from build123d import *

# Parameters (mm, degrees)
BOSS_EXTRUDE1_DEPTH = 1500
FILLET1_R           = 10
SKETCH2_R           = 37.5
CUT_EXTRUDE1_DEPTH  = 1540.683409016


with BuildPart() as part:
    # Sketch1 → Boss-Extrude1 (new body)
    with BuildSketch(Plane(origin=(0, 0, 0), x_dir=(1, 0, 0), z_dir=(0, 1, 0))):
        Polygon((175, 50), (300, 50), (300, 0), (0, 0), (0, 50), (125, 50), (125, 250), (0, 250), (0, 300), (300, 300), (300, 250), (175, 250), align=None)
    extrude(amount=BOSS_EXTRUDE1_DEPTH)

    # Fillet1
    fillet1_edges = [part.edges().sort_by_distance(p)[0] for p in [
        (125, 750, -50),
        (125, 750, -250),
        (175, 750, -250),
        (175, 750, -50),
    ]]
    fillet(fillet1_edges, radius=FILLET1_R)

    # Sketch2 → Cut-Extrude1 (cut, through all)
    with BuildSketch(Plane.ZY.offset(-125)):
        with Locations((-150, 1400)):
            Circle(SKETCH2_R)
        with Locations((-150, 1000)):
            Circle(SKETCH2_R)
    extrude(amount=-CUT_EXTRUDE1_DEPTH, mode=Mode.SUBTRACT)


solid = part.part
Read the model definition and answer for the solid it produces. Units are mm, in the model's axes. A direction names the side the tool comes from. Round coordinates to 2 decimals unless told otherwise and drop trailing zeros. Order: outer loops, then holes, each group sorted by start corner. A loop starts at its lowest first (then second) coordinate and runs counter-clockwise, first axis right, second up. Notation, with made-up numbers: (-15, 27.5) - (38, 27.5) arc R11 cw to (38, 33.5) - close; hole circle Ø11 at (7.25, 21.5). An arc over 180 degrees is marked (long way). Use one line per item in the form item = value. Start each with the question number.
(1) The part is cut by section D-D (y = 580). Give the vertices of the cut face in (x, z).
(2) Determine the mould class of faces 1 (the face through (152, 1500, -185)), 2 (the face through (242, 740, -50)), 3 (the face through (149.65, 966.73, -132.7)) for opening direction Y: +Y half, -Y half, draft (parallel to the pull), parting line (faces both ways), or undercut.
(3) For faces 4 (the face through (58, 740, -250)), 5 (the face through (0, 740, -275)), 6 (the face through (175, 740, -151)), determine the directions among +Z, -Z, +X, -X, +Y, -Y from which every point of the face is accessible in a straight line to the end or side of a thin tool.
(4) The part is cut by section C-C (z = -150). Give the vertices of the cut face in (x, y), then the cut area to 3 significant figures.
(5) The part is cut by section A-A (x = 262). Give the vertices of the cut face in (y, z).
(6) Flat-ended cylindrical pins translate along their axes: pin 1 Ø6 at (y, z) = (675.5, -171) entering from +X; pin 2 Ø6 at (y, z) = (1156, -55.5) entering from -X. Find the tip coordinate at first contact, or state that the pin passes through.
(7) The part is cut by section B-B (y = 1000). Give the vertices of the cut face in (x, z), then the cut area to 3 significant figures.
(8) Find the intervals of material crossed by line 1 along Y through (x, z) = (140, -150); line 2 along Z through (x, y) = (282.5, 388); line 3 along X through (y, z) = (1359, -98), in increasing order. Write a range as from..to.
Checked values:
q1.outline = (0, -300) - (300, -300) - (300, -250) - (185, -250) arc R10 cw to (175, -240) - (175, -60) arc R10 cw to (185, -50) - (300, -50) - (300, 0) - (0, 0) - (0, -50) - (115, -50) arc R10 cw to (125, -60) - (125, -240) arc R10 cw to (115, -250) - (0, -250) - close
q2.face_1 = +Y half
q2.face_2 = draft
q2.face_3 = undercut
q3.face_4 = -X, +Y, -Y
q3.face_5 = +Z, -Z, -X, +Y, -Y
q3.face_6 = +X, +Y, -Y
q4.outline = (125, 0) - (175, 0) - (175, 962.5) - (125, 962.5) - close; (125, 1037.5) - (175, 1037.5) - (175, 1362.5) - (125, 1362.5) - close; (125, 1437.5) - (175, 1437.5) - (175, 1500) - (125, 1500) - close
q4.area = 67,500 mm^2
q5.outline = (0, -300) - (1500, -300) - (1500, -250) - (0, -250) - close; (0, -50) - (1500, -50) - (1500, 0) - (0, 0) - close
q6.pin_1 = 175
q6.pin_2 = 121.61
q7.outline = (0, -300) - (300, -300) - (300, -250) - (185, -250) arc R10 cw to (175, -240) - (175, -187.5) - (125, -187.5) - (125, -240) arc R10 cw to (115, -250) - (0, -250) - close; (0, -50) - (115, -50) arc R10 cw to (125, -60) - (125, -112.5) - (175, -112.5) - (175, -60) arc R10 cw to (185, -50) - (300, -50) - (300, 0) - (0, 0) - close
q7.area = 36,300 mm^2
q8.line_1 = 0..962.5, 1037.5..1362.5, 1437.5..1500
q8.line_2 = -300..-250, -50..0
q8.line_3 = 125..175
